For this review, take the finished solid that the model builds, in its own axes (mm). Face numbers are marked on the shaded views. Give positions to 0.01 mm unless a question says otherwise; leave off trailing zeros. Use CSV: the item, a comma, the result in double quotes. Start each with the question number.
1. To check wall thickness, follow line 1 (X direction, y = 19, z = 41.5); line 2 (Z direction, x = 23, y = 14.5); line 3 (Z direction, x = 87, y = 16.5). State the ranges of each line that lie inside material, in increasing order. Write a range as [from, to].
2. Take a section at A-A, the plane y = 13. State how many separate pieces and enclosed holes the cut face has, and give its area (3 significant figures).
3. Insertion check: P1, Ø8, axis at x = -7.5, z = -111.5, coming from the +Y side; P2, Ø1, axis at x = 33, y = 31, coming from the +Z side. Each pin has a flat end and moves straight along its axis. Give the tip position at first contact, or say it passes through.
4. The part is to be moulded in two halves that separate along Z. For the marked faces 1, 2 and 3, say which applies: pulls with the +Z half, pulls with the -Z half, needs draft (parallel to the pull), parting line crosses it, or undercut.
from build123d import *

# Parameters (mm, degrees)
EXTRUDE_1_DEPTH     = 145
CUT_EXTRUDE_1_DEPTH = 150
CUT_EXTRUDE_2_DEPTH = 150
SHELL_1_T           = 3
CUT_EXTRUDE_4_DEPTH = 3
SKETCH_13_W         = 284
SKETCH_13_H         = 300
CUT_EXTRUDE_5_DEPTH = 3
CUT_EXTRUDE_6_DEPTH = 3


with BuildPart() as part:
    # 草图4 → 凸台-拉伸1 (new, symmetric)
    with BuildSketch(Plane(origin=(0, 0, 0), x_dir=(0, 0, -1), z_dir=(1, 0, 0))):
        Polygon((-148.47826087, 0), (157.52173913, 0), (157.52173913, 25), (145.02173913, 46.650635095), (-148.47826087, 30), align=None)
    extrude(amount=EXTRUDE_1_DEPTH, both=True)

    # 草图5 → 切除-放样1 section 0
    with BuildSketch(Plane(origin=(0, 74.458913868, -128.966621895), x_dir=(-1, 0, 0), z_dir=(0, 0.500000000000004, -0.8660254037844364))):
        with BuildLine():
            Line((-145, -47.110234471), (-85, -32.110234471))
            Line((-85, -32.110234471), (-145, -32.110234471))
            Line((-145, -32.110234471), (-145, -47.110234471))
        make_face()
    # 草图6 → 切除-放样1 section 1
    with BuildSketch(Plane.XY.offset(148.47826087)):
        with BuildLine():
            Line((145, 30), (120, 30))
            Line((120, 30), (145, 25))
            Line((145, 25), (145, 30))
        make_face()
    loft(mode=Mode.SUBTRACT)

    # 草图7 → 切除-放样2 section 0
    with BuildSketch(Plane(origin=(0, 74.458913868, -128.966621895), x_dir=(-1, 0, 0), z_dir=(0, 0.500000000000004, -0.8660254037844364))):
        with BuildLine():
            Line((145, -32.110234471), (85, -32.110234471))
            Line((85, -32.110234471), (145, -47.110234471))
            Line((145, -47.110234471), (145, -32.110234471))
        make_face()
    # 草图8 → 切除-放样2 section 1
    with BuildSketch(Plane.XY.offset(148.47826087)):
        with BuildLine():
            Line((-120, 30), (-145, 30))
            Line((-145, 30), (-145, 25))
            Line((-145, 25), (-120, 30))
        make_face()
    loft(mode=Mode.SUBTRACT)

    # 草图9 → 切除-拉伸1 (cut, symmetric)
    with BuildSketch(Plane(origin=(0, 0, 0), x_dir=(0, 0, -1), z_dir=(1, 0, 0))):
        Polygon((-148.47826087, 25), (-137.542379964, 30.620406686), (-148.47826087, 30), align=None)
    extrude(amount=CUT_EXTRUDE_1_DEPTH, both=True, mode=Mode.SUBTRACT)

    # 草图10 → 切除-拉伸2 (cut, symmetric)
    with BuildSketch(Plane(origin=(0, 0, 0), x_dir=(0, 0, -1), z_dir=(1, 0, 0))):
        Polygon((152.52173913, 33.660254038), (130.045819319, 45.801031769), (145.02173913, 46.650635095), align=None)
    extrude(amount=CUT_EXTRUDE_2_DEPTH, both=True, mode=Mode.SUBTRACT)

    # 抽壳1 (no face opened: a closed hollow body)
    add(offset(amount=-SHELL_1_T, mode=Mode.PRIVATE), mode=Mode.SUBTRACT)

    # 草图12 → 切除-拉伸4 (cut)
    with BuildSketch(Plane.XY.offset(148.47826087)):
        with BuildLine():
            Line((-76.5, 21.5), (-76.5, 3.5))
            ThreePointArc((-76.5, 3.5), (-78.5, 1.5), (-80.5, 3.5))
            Line((-80.5, 3.5), (-80.5, 21.5))
            ThreePointArc((-80.5, 21.5), (-78.5, 23.5), (-76.5, 21.5))
        make_face()
        with BuildLine():
            Line((-101.5, 21.5), (-101.5, 3.5))
            ThreePointArc((-101.5, 3.5), (-103.5, 1.5), (-105.5, 3.5))
            Line((-105.5, 3.5), (-105.5, 21.5))
            ThreePointArc((-105.5, 21.5), (-103.5, 23.5), (-101.5, 21.5))
        make_face()
        with BuildLine():
            Line((76.5, 21.5), (76.5, 3.5))
            ThreePointArc((76.5, 3.5), (78.5, 1.5), (80.5, 3.5))
            Line((80.5, 3.5), (80.5, 21.5))
            ThreePointArc((80.5, 21.5), (78.5, 23.5), (76.5, 21.5))
        make_face()
        with BuildLine():
            Line((101.5, 21.5), (101.5, 3.5))
            ThreePointArc((101.5, 3.5), (103.5, 1.5), (105.5, 3.5))
            Line((105.5, 3.5), (105.5, 21.5))
            ThreePointArc((105.5, 21.5), (103.5, 23.5), (101.5, 21.5))
        make_face()
    extrude(amount=-CUT_EXTRUDE_4_DEPTH, mode=Mode.SUBTRACT)

    # 草图13 → 切除-拉伸5 (cut)
    with BuildSketch(Plane.XZ):
        with Locations((0, -4.52173913)):
            Rectangle(SKETCH_13_W, SKETCH_13_H)
    extrude(amount=-CUT_EXTRUDE_5_DEPTH, mode=Mode.SUBTRACT)

    # 草图14 → 切除-拉伸6 (cut)
    with BuildSketch(Plane(origin=(0, 0, -157.52173913), x_dir=(-1, 0, 0), z_dir=(0, 0, -1))):
        with BuildLine():
            Line((-46.5, 19.5), (-46.5, 4.5))
            ThreePointArc((-46.5, 4.5), (-49, 2), (-51.5, 4.5))
            Line((-51.5, 4.5), (-51.5, 19.5))
            ThreePointArc((-51.5, 19.5), (-49, 22), (-46.5, 19.5))
        make_face()
        with BuildLine():
            Line((-82.454286499, 19.5), (-82.454286499, 4.5))
            ThreePointArc((-82.454286499, 4.5), (-85, 1.954286499), (-87.545713501, 4.5))
            Line((-87.545713501, 4.5), (-87.545713501, 19.5))
            ThreePointArc((-87.545713501, 19.5), (-85, 22.045713501), (-82.454286499, 19.5))
        make_face()
        with BuildLine():
            Line((46.5, 19.5), (46.5, 4.5))
            ThreePointArc((46.5, 4.5), (49, 2), (51.5, 4.5))
            Line((51.5, 4.5), (51.5, 19.5))
            ThreePointArc((51.5, 19.5), (49, 22), (46.5, 19.5))
        make_face()
        with BuildLine():
            Line((82.454286499, 19.5), (82.454286499, 4.5))
            ThreePointArc((82.454286499, 4.5), (85, 1.954286499), (87.545713501, 4.5))
            Line((87.545713501, 4.5), (87.545713501, 19.5))
            ThreePointArc((87.545713501, 19.5), (85, 22.045713501), (82.454286499, 19.5))
        make_face()
    extrude(amount=-CUT_EXTRUDE_6_DEPTH, mode=Mode.SUBTRACT)


solid = part.part
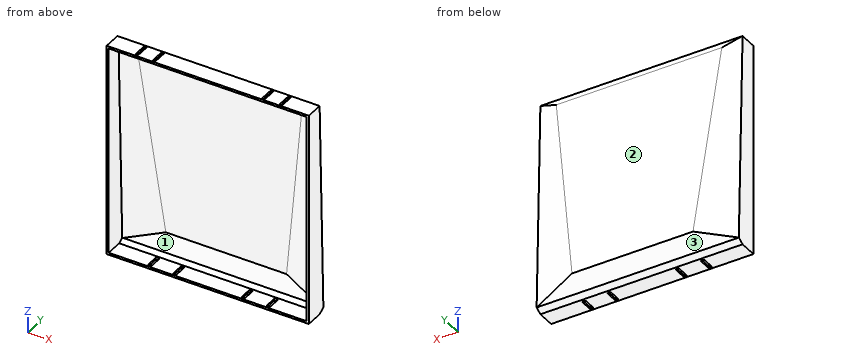
Result set:
1,line 1,"[-145, -142], [142, 145]"
1,line 2,"[-157.52, -154.52], [145.48, 148.48]"
1,line 3,"[145.48, 148.48]"
2,separate pieces,"8"
2,enclosed holes,"0"
2,area,"3,430 mm2"
3,P1,"y = 44.98"
3,P2,"z = 137.78"
4,face 1,"undercut"
4,face 2,"pulls with the +Z half"
4,face 3,"pulls with the -Z half"
